from build123d import *

# Parameters (mm, degrees)
SKETCH_1_W          = 116
SKETCH_1_H          = 144
EXTRUDE_1_DEPTH     = 120
SKETCH_2_R          = 12
EXTRUDE_3_DEPTH     = 32
SKETCH_6_W          = 72
SKETCH_6_H          = 40
CUT_EXTRUDE_1_DEPTH = 182.76908428
CUT_EXTRUDE_3_REACH = 202.848
CUT_EXTRUDE_4_REACH = 247.797
SKETCH_10_R         = 16
CUT_EXTRUDE_5_DEPTH = 201.848142751
SKETCH_11_R         = 27
CUT_EXTRUDE_6_DEPTH = 22


with BuildPart() as part:
    # 草图1 → 凸台-拉伸1 (new body)
    with BuildSketch(Plane(origin=(0, 0, 0), x_dir=(1, 0, 0), z_dir=(0, 1, 0))):
        Rectangle(SKETCH_1_W, SKETCH_1_H)
    extrude(amount=-EXTRUDE_1_DEPTH)

    # 草图2 → 凸台-拉伸3 (add)
    with BuildSketch(Plane(origin=(0, 0, 0), x_dir=(1, 0, 0), z_dir=(0, 1, 0))):
        with BuildLine():
            Line((-58, 42), (-102.069345964, 42))
            ThreePointArc((-102.069345964, 42), (-144.069345964, 0), (-102.069345964, -42))
            Line((-102.069345964, -42), (-58, -42))
            Line((-58, -42), (-58, 42))
        make_face()
        with Locations(Location((-102.069345964, 0, 0), (0, 0, 270))):
            Circle(SKETCH_2_R, mode=Mode.SUBTRACT)
    extrude_3 = extrude(amount=-EXTRUDE_3_DEPTH)

    # 草图6 → 切除-拉伸1 (cut, through all)
    with BuildSketch(Plane.ZY.offset(58)):
        with Locations((36, -68)):
            Rectangle(SKETCH_6_W, SKETCH_6_H)
    extrude(amount=-CUT_EXTRUDE_1_DEPTH, mode=Mode.SUBTRACT)

    # 草图8 → 切除-拉伸3 (cut, up to next)
    with BuildSketch(Plane.XZ.offset(120), mode=Mode.PRIVATE) as cut_extrude_3_sk1:
        Polygon((-38, 72), (-58, 37), (-58, 72), align=None)
    cut_extrude_3_tool1 = extrude(cut_extrude_3_sk1.sketch, amount=-CUT_EXTRUDE_3_REACH, mode=Mode.PRIVATE) & part.part
    cut_extrude_3 = cut_extrude_3_tool1.solids().sort_by_distance((-51.333333, -120, 60.333333))[0]
    add(cut_extrude_3, mode=Mode.SUBTRACT)

    # 镜向1: 凸台-拉伸3, 切除-拉伸3 across plane
    add(extrude_3.mirror(Plane(origin=(0, 0, 0), x_dir=(0, 0, 1), z_dir=(1, 0, 0))))
    add(cut_extrude_3.mirror(Plane(origin=(0, 0, 0), x_dir=(0, 0, 1), z_dir=(1, 0, 0))), mode=Mode.SUBTRACT)

    # 草图9 → 切除-拉伸4 (cut, up to next)
    with BuildSketch(Plane.ZY.offset(58), mode=Mode.PRIVATE) as cut_extrude_4_sk1:
        Polygon((-72, -100), (-52, -120), (-72, -120), align=None)
    cut_extrude_4_tool1 = extrude(cut_extrude_4_sk1.sketch, amount=-CUT_EXTRUDE_4_REACH, mode=Mode.PRIVATE) & part.part
    add(cut_extrude_4_tool1.solids().sort_by_distance((-58, -113.333333, -65.333333))[0], mode=Mode.SUBTRACT)

    # 草图10 → 切除-拉伸5 (cut, through all)
    with BuildSketch(Plane(origin=(0, 0, 0), x_dir=(1, 0, 0), z_dir=(0, 1, 0))):
        with Locations(Location((0, -30, 0), (0, 0, 270))):
            Circle(SKETCH_10_R)
    extrude(amount=-CUT_EXTRUDE_5_DEPTH, mode=Mode.SUBTRACT)

    # 草图11 → 切除-拉伸6 (cut)
    with BuildSketch(Plane.XZ.offset(120)):
        with Locations(Location((0, 30, 0), (0, 0, 270))):
            Circle(SKETCH_11_R)
    extrude(amount=-CUT_EXTRUDE_6_DEPTH, mode=Mode.SUBTRACT)


solid = part.part
Build history of the part. All positions in model axes, mm. A direction names the side the tool comes from. Round coordinates to 2 decimals unless told otherwise and drop trailing zeros. Write each loop counter-clockwise with the first axis right and the second up, starting at its lowest first coordinate (ties: lowest second). Pieces come first, ordered by that corner, then holes. Notation, with made-up numbers: (-21, -11) - (18, -11) arc R6 cw to (18, -4) - close; hole circle Ø9 at (55.5, 59). An arc over 180 degrees is marked (long way). One line per question, with ' | ' between items.
1. Band-saw the part on D-D, the plane z = 30. Write the cut outline in (x, y).
Results are:
outline: (-131.46, -32) - (-58, -32) - (-58, -48) - (-16, -48) - (-16, 0) - (-131.46, 0) - close; (-58, -120) - (-27, -120) - (-27, -98) - (-16, -98) - (-16, -88) - (-58, -88) - close; (16, -98) - (27, -98) - (27, -120) - (58, -120) - (58, -88) - (16, -88) - close; (16, -48) - (58, -48) - (58, -32) - (131.46, -32) - (131.46, 0) - (16, 0) - close
2. Drill centre lines: line 1 along X through (y, z) = (-7, 0); line 2 along X through (y, z) = (-38, 30); line 3 along Z through (x, y) = (-39.5, -49.5). Where is each one in solid material? Low to high. Write a range as from..to.
Results are:
line 1: -144.07..-114.07, -90.07..90.07, 114.07..144.07 | line 2: -58..-16, 16..58 | line 3: -72..0
3. Tool access for faces 1 (the face through (92, -32, 9)), 2 (the face through (-80, -16, 42)), 3 (the face through (80, -16, 42)): list every direction of +Z, -Z, +X, -X, +Y, -Y with a clear straight run to the whole face (end or side of a thin tool).
Results are:
face 1: +Z, -Z, +X, -Y | face 2: +Z, -X, +Y, -Y | face 3: +Z, +X, +Y, -Y
4. Band-saw the part on C-C, the plane z = -17. Write the cut outline in (x, y).
Results are:
outline: (-140.48, -32) - (-58, -32) - (-58, -120) - (58, -120) - (58, -32) - (140.48, -32) - (140.48, 0) - (-140.48, 0) - close
5. Band-saw the part on B-B, the plane x = 0. Write the cut outline in (y, z).
Results are:
outline: (-120, -52) - (-100, -72) - (0, -72) - (0, 14) - (-48, 14) - (-48, 0) - (-88, 0) - (-88, 14) - (-98, 14) - (-98, 3) - (-120, 3) - close; (-120, 57) - (-98, 57) - (-98, 46) - (-88, 46) - (-88, 72) - (-120, 72) - close; (-48, 46) - (0, 46) - (0, 72) - (-48, 72) - close
6. Band-saw the part on A-A, the plane y = -17.5. Write the cut outline in (x, z).
Results are:
outline: (-102.07, -42) - (-58, -42) - (-58, -72) - (58, -72) - (58, -42) - (102.07, -42) arc R42 ccw to (102.07, 42) - (58, 42) - (58, 72) - (-58, 72) - (-58, 42) - (-102.07, 42) arc R42 ccw to start; hole circle Ø24 at (-102.07, 0); hole circle Ø32 at (0, 30); hole circle Ø24 at (102.07, 0)
7. Mould opens along Z. For faces 4 (the face through (-12, -98, 18)), 5 (the face through (-1, -110, -62)), 6 (the face through (-9.736, -23.664, 17.303)), 7 (the face through (58, -59, -15)) say: released by +Z, released by -Z, zero draft, split by the parting line, or undercut.
Results are:
face 4: undercut | face 5: released by -Z | face 6: undercut | face 7: zero draft
8. Drop flat-ended pins along their axis: pin 1 Ø25 at (x, z) = (83, 7.5) entering from -Y; pin 2 Ø3 at (y, z) = (-99.5, -17) entering from +X; pin 3 Ø14.5 at (x, z) = (-102.07, 0) entering from +Y; pin 4 Ø9.5 at (x, y) = (-86, -16) entering from -Z. Give the stop position or say it passes through.
Results are:
pin 1: y = -32 | pin 2: x = 58 | pin 3: through | pin 4: z = -42
